```python
from build123d import *

# Parameters (mm, degrees)
EXTRUDE_1_DEPTH              = 100
SKETCH_2_R                   = 9
CUT_EXTRUDE_1_DEPTH          = 100
HOLE_WIZARD_M3_3_D           = 2.5
HOLE_WIZARD_M3_3_CSINK_D     = 3.05
HOLE_WIZARD_M3_3_CSINK_ANGLE = 90
HOLE_WIZARD_M3_4_D           = 2.5
HOLE_WIZARD_M3_4_CSINK_D     = 3.05
HOLE_WIZARD_M3_4_CSINK_ANGLE = 90


with BuildPart() as part:
    # 草图1 → 凸台-拉伸1 (new body)
    with BuildSketch(Plane.XY):
        with BuildLine():
            Line((0, 0), (5, 0))
            Line((5, 0), (5, 540))
            ThreePointArc((5, 540), (0, 575.291616466), (-5, 540))
            Line((-5, 540), (-5, 0))
            Line((-5, 0), (0, 0))
        make_face()
    extrude(amount=EXTRUDE_1_DEPTH)

    # 草图2 → 切除-拉伸1 (cut)
    with BuildSketch(Plane.XY.offset(100)):
        with Locations((0, 557.291616466)):
            Circle(SKETCH_2_R)
    extrude(amount=-CUT_EXTRUDE_1_DEPTH, mode=Mode.SUBTRACT)

    # M3 螺纹孔3 (through all)
    with Locations(Plane(origin=(5, 500, 49.938905555), x_dir=(0, 0, 1), z_dir=(1, 0, 0))):
        with Locations((0, 0)):
            CounterSinkHole(HOLE_WIZARD_M3_3_D / 2, HOLE_WIZARD_M3_3_CSINK_D / 2, counter_sink_angle=HOLE_WIZARD_M3_3_CSINK_ANGLE)

    # M3 螺纹孔4 (through all)
    with Locations(Plane(origin=(5, 480, 49.890282126), x_dir=(0, 0, 1), z_dir=(1, 0, 0))):
        with Locations((0, 0)):
            CounterSinkHole(HOLE_WIZARD_M3_4_D / 2, HOLE_WIZARD_M3_4_CSINK_D / 2, counter_sink_angle=HOLE_WIZARD_M3_4_CSINK_ANGLE)


solid = part.part
```
Could you check a few things on this model? Use its own coordinates, in mm. A direction names the side the tool comes from. Give positions to 0.01 mm unless a question says otherwise; leave off trailing zeros. Loops run counter-clockwise (first coordinate to the right, second up) from the corner with the lowest first, then second, coordinate; pieces in that order, holes last. Notation, with made-up numbers: (38, -4) - (47, -4) arc R17 ccw to (47, 11) - close; hole circle Ø1 at (61, 53.5). An arc over 180 degrees is marked (long way). Use one line per item in the form item = value.
1. I want a section at C-C (y = 117). Please give me the cut outline in (x, z), and give its area (3 significant figures).
Response values:
outline = (-5, 0) - (5, 0) - (5, 100) - (-5, 100) - close
area = 1,000 mm²
2. I need wall thicknesses on probe 1 along Y at (x, z) = (0, 72); probe 2 along X at (y, z) = (505, 32); probe 3 along Z at (x, y) = (1.25, 500). Which ranges of each line are inside material? Lowest first, please.
Response values:
probe_1 = 0 to 548.29, 566.29 to 575.29
probe_2 = -5 to 5
probe_3 = 0 to 48.69, 51.19 to 100
3. I want a section at B-B (z = 25.5). Please give me the cut outline in (x, y), and give its area (3 significant figures).
Response values:
outline = (-5, 0) - (5, 0) - (5, 540) arc R18 ccw (long way) to (-5, 540) - close; hole circle Ø18 at (0, 557.29)
area = 6,160 mm²
4. I want a section at A-A (x = 0). Please give me the cut outline in (y, z).
Response values:
outline = (0, 0) - (548.29, 0) - (548.29, 100) - (0, 100) - close; (566.29, 0) - (575.29, 0) - (575.29, 100) - (566.29, 100) - close; hole circle Ø2.5 at (480, 49.89); hole circle Ø2.5 at (500, 49.94)
5. Thinking about a two-plate mould opening in Y: for faces 1 (the face through (0, 356, 0)), 2 (the face through (-1.951, 548.506, 50.7)), 3 (the face through (0.721, 575.277, 49.3)), which applies, released by +Y, released by -Y, zero draft, split by the parting line, or undercut?
Response values:
face_1 = zero draft
face_2 = undercut
face_3 = split by the parting line
6. On a 3-axis mill with a long thin cutter (end or side, diameter ignored), from which of +Z, -Z, +X, -X, +Y, -Y can I reach the whole of each face in a straight line? I mean faces 4 (the face through (0, 356, 100)), 5 (the face through (5, 266, 49)), 6 (the face through (-5, 274, 49)). Say none if no direction works.
Response values:
face_4 = +Z, +X, -X, +Y, -Y
face_5 = +Z, -Z, +X, -Y
face_6 = +Z, -Z, -X, -Y
7. I'm going to push flat-ended pins straight in: pin 1 Ø5 at (y, z) = (178.5, 17.5) entering from +X; pin 2 Ø2 at (y, z) = (480, 49.89) entering from +X; pin 3 Ø4 at (y, z) = (264, 62.5) entering from -X; pin 4 Ø3 at (x, z) = (-12.5, 24.5) entering from +Y. Where does each tip first touch, or does it pass through?
Response values:
pin_1 = 5
pin_2 = through
pin_3 = -5
pin_4 = 571.54
